```python
from build123d import *

# Parameters (mm, degrees)
F0_R     = 2
F0_R_2   = 1.125
F1_DEPTH = 9
F0_R_3   = 4
F2_DEPTH = 0.75
F3_SIZE  = 0.5


with BuildPart() as f1:
    # F0 (on Top) → F1 (new body)
    with BuildSketch(Plane.XY):
        Circle(F0_R)
        Circle(F0_R_2, mode=Mode.SUBTRACT)
    extrude(amount=F1_DEPTH)

    # F0 (on Top) → F2 (join)
    with BuildSketch(Plane.XY):
        Circle(F0_R_3)
        Circle(F0_R, mode=Mode.SUBTRACT)
        Circle(F0_R)
        Circle(F0_R_2, mode=Mode.SUBTRACT)
    extrude(amount=-F2_DEPTH)

    # F3
    f3_edges = [f1.edges().sort_by_distance(p)[0] for p in [
        (-1.125, 0, 9),
        (1.125, 0, 4.125),
        (-1.125, 0, -0.75),
        (-4, 0, -0.75),
    ]]
    chamfer(f3_edges, length=F3_SIZE)


solid = f1.part
```
Geometry check sheet. Reference: the model listing, model coordinates, mm. A direction names the side the tool comes from. Coordinates: 2 decimals unless noted, no trailing zeros. Order: outer loops, then holes, each group sorted by start corner. A loop starts at its lowest first (then second) coordinate and runs counter-clockwise, first axis right, second up. Notation, with made-up numbers: (81, 6.5) - (136, 6.5) arc R23 ccw to (136, 33.5) - close; hole circle Ø4 at (-35.5, 1.5). An arc over 180 degrees is marked (long way). Answer as a JSON object with one key per item and string values. Group by question number.
Item 1: Sectioned sample at C-C, the plane z = 4. Record the cut outline in (x, y) (3 decimals), and give its area (3 significant figures).
Item 2: Tool access check on faces 1 (the face through (0, -2, 4)), 2 (the face through (1, -2, -0.75)). Record the directions out of +Z, -Z, +X, -X, +Y, -Y that give a thin tool (end or side, any length) a straight path to the whole face; none if there is none.
Item 3: Scan lines: probe 1 along Y at (x, z) = (0, -0.05) (3 decimals); probe 2 along Z at (x, y) = (-0.5, -2.25); probe 3 along Y at (x, z) = (0, 6.25) (3 decimals). Record each from-to range of solid material in increasing order.
Item 4: Sectioned sample at A-A, the plane x = 0. Record the cut outline in (y, z) (3 decimals).
Item 5: Depth check by flat-ended pin: pin 1 Ø2.5 at (x, y) = (0, 0) entering from -Z (3 decimals); pin 2 Ø1 at (x, z) = (-1.5, 2) entering from -Y. Enter the tip coordinate at first touch or a pass-through.
Resolved:
{
 "1": {"outline": "circle Ø4 at (0, 0); hole circle Ø2.25 at (0, 0)", "area": "8.59 mm^2"},
 "2": {"face 1": "+Z", "face 2": "-Z, +X, -X, +Y, -Y"},
 "3": {"probe 1": "-4 to -1.125, 1.125 to 4", "probe 2": "-0.75 to 0", "probe 3": "-2 to -1.125, 1.125 to 2"},
 "4": {"outline": "(-4, -0.25) - (-3.5, -0.75) - (-1.625, -0.75) - (-1.125, -0.25) - (-1.125, 8.5) - (-1.625, 9) - (-2, 9) - (-2, 0) - (-4, 0) - close; (1.125, -0.25) - (1.625, -0.75) - (3.5, -0.75) - (4, -0.25) - (4, 0) - (2, 0) - (2, 9) - (1.625, 9) - (1.125, 8.5) - close"},
 "5": {"pin 1": "z = -0.375", "pin 2": "y = -1.73"}
}
